Geometry: final body of the model. Coordinates: model frame, mm. Face numbers are marked on the shaded views. A direction names the side the tool comes from. Give positions to 0.01 mm unless a question says otherwise; leave off trailing zeros. Write each loop counter-clockwise with the first axis right and the second up, starting at its lowest first coordinate (ties: lowest second). Pieces come first, ordered by that corner, then holes.
Q1. Reachability of the marked faces 1, 2 and 3 from +Z, -Z, +X, -X, +Y, -Y: full face, straight path, thin tool, end or side. Return the list, or none.
Q2. Pin query (flat end, axial travel): pin 1 (5 mm diameter, centred on x = 21.5, y = -31.5, fed in from +Z); pin 2 (1.5 mm diameter, centred on x = 27.5, y = -77.5, fed in from -Z); pin 3 (1 mm diameter, centred on x = 20, y = -66, fed in from -Z). Return the tip coordinate at first contact, or that it passes through.
Q3. Cut plane A-A on x = 25.5. Return the cut outline in (y, z).
Q4. Line query: L1, parallel to Z at x = 13.5, y = -85; L2, parallel to Y at x = -9, z = -48.5; L3, parallel to X at y = -33.5, z = 11. Output: solid intervals per line, ascending.
Q5. Cut plane D-D on x = -14. Return the cut outline in (y, z).
Q6. Cut plane C-C on y = -52.5. Return the cut outline in (x, z), plus the area to 3 significant figures.
Q7. Cut plane B-B on z = -16. Return the cut outline in (x, y).
Autodesk Inventor part; units mm, degrees
ref_plane "Work Plane1" through (0, -73.5, -54.5) normal (0, 1, 0) x (1, 0, 0)
ref_plane "YZ Plane" through (0, 0, 0) normal (1, 0, 0) x (0, 1, 0)
ref_plane "XZ Plane" through (0, 0, 0) normal (0, 1, 0) x (-1, 0, 0)
sketch "Sketch1" plane through (0, 0, 0) normal (1, 0, 0) x (0, 1, 0)
  circle A0 centre (0, 0) radius 22.5
  line L0 (0, 22.5) -> (-50, 22.5)
  line L1 (-50, 22.5) -> (-50, -54.5)
  line L2 (-50, -54.5) -> (11.1665, -19.5335)
  dimension "d0" = 45
  dimension "d1" = 50
  dimension "d2" = 77
extrude "Extrusion1" add sketch "Sketch1" along normal blind 28
sketch "Sketch2" plane through (0, -50, -54.5) normal (0, -1, 0) x (1, 0, 0)
  circle A0 centre (14, 38.5) radius 45
  line L0 (0, 77) -> (28, 77)
  line L1 (0, 77) -> (0, 0)
  point P0 (0, 54.5)
  point P1 (14, 77)
  point P2 (0, 38.5)
  dimension "d5" = 90
extrude "Extrusion2" add sketch "Sketch2" along normal blind 47
sketch "Sketch3" plane through (14, -97, -16) normal (0, -1, 0) x (1, 0, 0)
  circle A0 centre (0, 0) radius 45
  circle A1 centre (0, 0) radius 40
  line L0 (0, 0) -> (-45, 0) construction
  line L1 (0, 0) -> (-38.9711, 22.5) construction
  line L2 (0, 0) -> (-38.9711, -22.5) construction
  line L3 (-34.641, 20) -> (-24.3333, 37.8536)
  line L4 (-34.641, -20) -> (-24.3333, -37.8536)
  point P0 (-14, 16)
  dimension "d14" = 80
  dimension "d15" = 30
extrude "Extrusion3" cut sketch "Sketch3" against normal through all contours L3 A1 L4 A0 picked at (-30.1132, -30.0405)
ref_plane "Work Plane1" through (0, -73.5, -54.5) normal (0, 1, 0) x (1, 0, 0)
properties part number "hip_back"
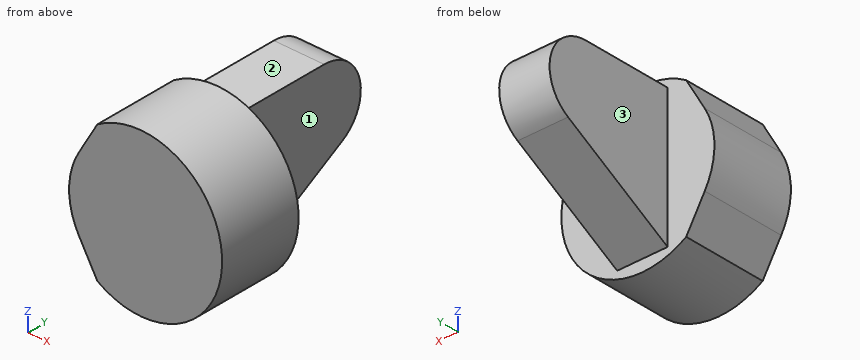
Data:
1. face 1: +Z, -Z, +X, +Y
1. face 2: +Z, +X, -X, +Y
1. face 3: +Z, -Z, -X, +Y
2. pin 1: stops at z = 22.5
2. pin 2: stops at z = -59.16
2. pin 3: stops at z = -60.66
3. outline: (-97, -59.51) - (-50, -59.51) - (-50, -54.5) - (11.17, -19.53) arc R22.5 ccw to (0, 22.5) - (-50, 22.5) - (-50, 27.51) - (-97, 27.51) - close
4. L1: z = -61 to 29
4. L2: y = -97 to -50
4. L3: x = 0 to 28
5. outline: (-97, -47.5) - (-50, -47.5) - (-50, 15.5) - (-97, 15.5) - close
6. outline: (-20.64, -36) - (-10.33, -53.85) arc R45 ccw (long way) to (-10.33, 21.85) - (-20.64, 4) arc R40 ccw to start
6. area: 6,000 mm2
7. outline: (-26, -97) - (59, -97) - (59, -50) - (28, -50) - (28, 15.82) - (0, 15.82) - (0, -50) - (-26, -50) - close
